Could you check a few things on this drawing? It's one solid part, dimensions in mm from its lowest x, y, z. Give positions to 0.01 mm unless a question says otherwise; leave off trailing zeros. Loops run counter-clockwise (first coordinate to the right, second up) from the corner with the lowest first, then second, coordinate; pieces in that order, holes last. Notation, with made-up numbers: M 88.25,56.25 L 102.25,56.25 A27 ccw 102.25,72.25 Z; hole C -36.75,-15.5 d5. An arc over 180 degrees is marked long. Return JSON: item names as keys, results as strings. Group by question number.
1. If we section it at A-A (z = 28.4): Write out the boundary of the cut face in (x, y), plus the area to 3 significant figures.
2. If we mould it in two halves opening along Z, with no side actions, what happens to the marked faces 1, 2 and 3? For each: +Z half, -Z half, draft (parallel to the pull), parting line (faces both ways), or undercut.
3. For pin 1 (4 mm diameter, centred on y = 10, z = 38.5, fed in from +X); pin 2 (5 mm diameter, centred on x = 27.5, y = 5, fed in from -Z); pin 3 (5 mm diameter, centred on x = 28.4, z = 52.15, fed in from +Y); pin 4 (1 mm diameter, centred on x = 23, y = 15, fed in from -Z), each with a flat end and sliding along its axis, tell me the tip position at first contact or that it passes through.
4. If we section it at B-B (x = 28.4): Write out the boundary of the cut face in (y, z), plus the area to 3 significant figures.
5. If we section it at D-D (z = 15): Write out the boundary of the cut face in (x, y), plus the area to 4 significant figures.
6. Please list where these lines run through material, in increasing order: line 1 (Z direction, x = 28.4, y = 2.7); line 2 (X direction, y = 2, z = 14); line 3 (Z direction, x = 28, y = 24.75).
7. If we section it at C-C (y = 2): Write out the boundary of the cut face in (x, z) (3 decimals), plus the area to 3 significant figures.
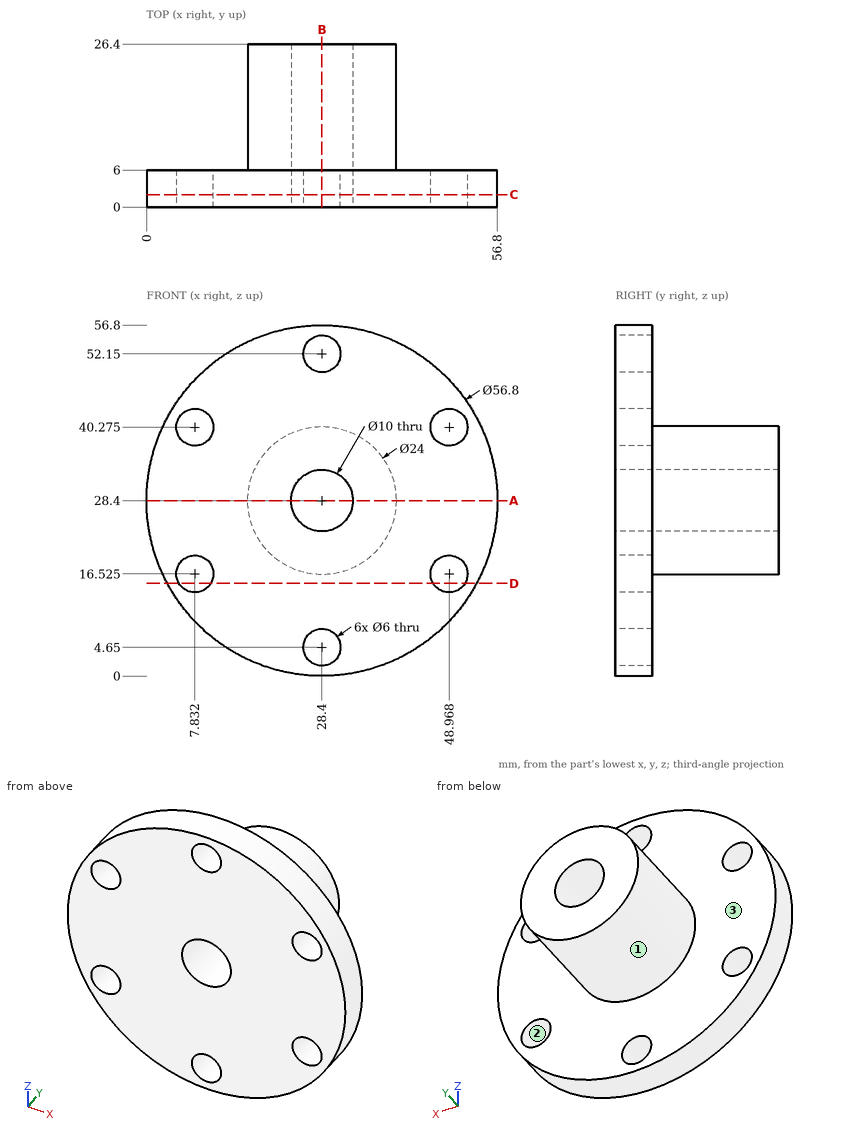
Answer:
{
 "1": {"outline": "M 0,0 L 23.4,0 L 23.4,26.4 L 16.4,26.4 L 16.4,6 L 0,6 Z; M 33.4,0 L 56.8,0 L 56.8,6 L 40.4,6 L 40.4,26.4 L 33.4,26.4 Z", "area": "566 mm²"},
 "2": {"face 1": "parting line", "face 2": "undercut", "face 3": "draft"},
 "3": {"pin 1": "stops at x = 37.25", "pin 2": "stops at z = 0", "pin 3": "passes through", "pin 4": "stops at z = 17.45"},
 "4": {"outline": "M 0,0 L 6,0 L 6,1.65 L 0,1.65 Z; M 0,7.65 L 6,7.65 L 6,16.4 L 26.4,16.4 L 26.4,23.4 L 0,23.4 Z; M 0,33.4 L 26.4,33.4 L 26.4,40.4 L 6,40.4 L 6,49.15 L 0,49.15 Z; M 0,55.15 L 6,55.15 L 6,56.8 L 0,56.8 Z", "area": "494 mm²"},
 "5": {"outline": "M 3.36,0 L 5.25,0 L 5.25,6 L 3.36,6 Z; M 10.42,0 L 46.38,0 L 46.38,6 L 10.42,6 Z; M 51.55,0 L 53.44,0 L 53.44,6 L 51.55,6 Z", "area": "238.5 mm²"},
 "6": {"line 1": "z = 0 to 1.65, 7.65 to 23.4, 33.4 to 49.15, 55.15 to 56.8", "line 2": "x = 3.92 to 6.21, 9.45 to 47.35, 50.59 to 52.88", "line 3": "z = 16.41 to 23.42, 33.38 to 40.39"},
 "7": {"outline": "C 28.4,28.4 d56.8; hole C 7.832,16.525 d6; hole C 7.832,40.275 d6; hole C 28.4,28.4 d10; hole C 28.4,4.65 d6; hole C 28.4,52.15 d6; hole C 48.968,16.525 d6; hole C 48.968,40.275 d6", "area": "2,290 mm²"}
}
